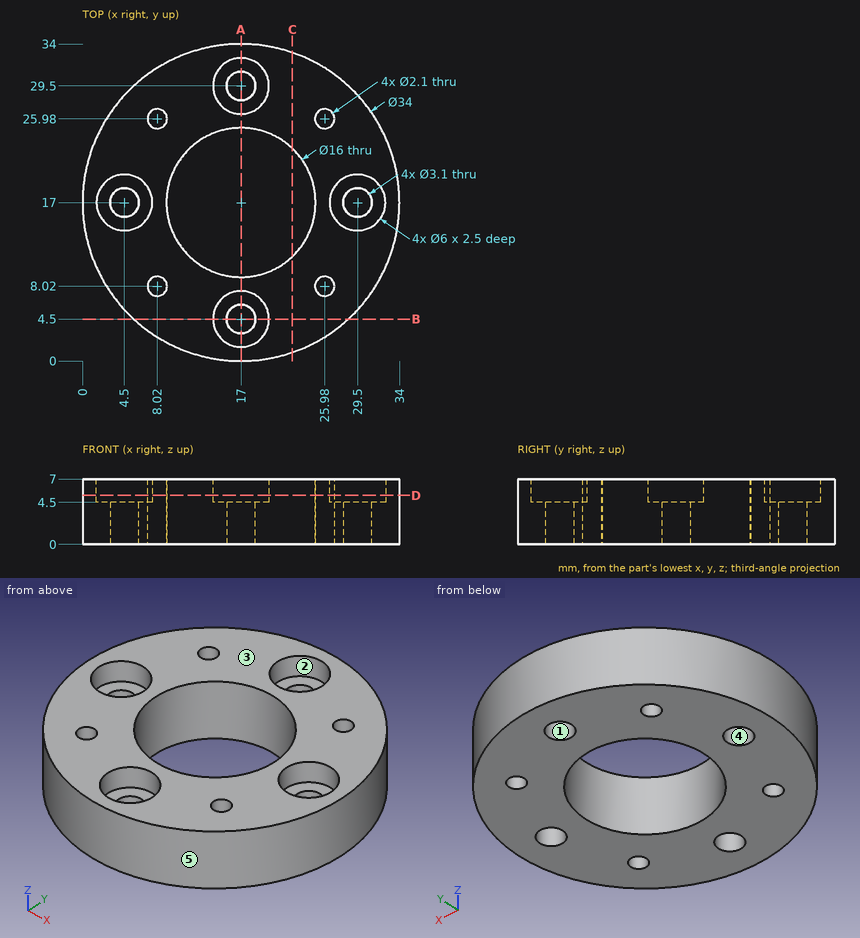
Answer from the drawing. Dimensions are ordinates in mm from the lowest x, y and z of the part. A direction names the side the tool comes from. Round coordinates to 2 decimals unless told otherwise and drop trailing zeros. Write each loop counter-clockwise with the first axis right and the second up, starting at its lowest first coordinate (ties: lowest second). Pieces come first, ordered by that corner, then holes.
1. The part is cut by section D-D, the plane z = 5.25. State how many separate pieces and enclosed holes the cut face has, then the cut area to 3 significant figures.
2. The part is cut by section A-A, the plane x = 17. Determine the outline of the cut face in (y, z).
3. Which of the six approach directions +Z, -Z, +X, -X, +Y, -Y give full straight-line access (tool end or side, diameter ignored) to the marked faces 1 and 2?
4. Straight lines are drawn through the part: L1, parallel to Y at x = 17, z = 1.05; L2, parallel to Y at x = 17, z = 5.25; L3, parallel to X at y = 19, z = 2.25. For each, find the intervals that lie inside material, in ascending order.
5. The part is cut by section B-B, the plane y = 4.5. Determine the outline of the cut face in (x, z).
6. Determine the mould class of the marked faces 3, 4 and 5 for opening direction Y: pulls with the +Y half, pulls with the -Y half, needs draft (parallel to the pull), parting line crosses it, or undercut.
7. Given pin 1 Ø12 at (x, y) = (6, 16) entering from -Z; pin 2 Ø1.9 at (x, y) = (25.98, 25.98) entering from +Z; pin 3 Ø4 at (x, y) = (29.5, 17) entering from +Z; pin 4 Ø3 at (x, z) = (23, 4) entering from -Y, each flat-ended and moving along its own axis, determine where each tip first touches the part or whether it passes through.
8. The part is cut by section C-C, the plane x = 22.5. Determine the outline of the cut face in (y, z).
Values:
1. separate pieces: 1
1. enclosed holes: 9
1. area: 580 mm2
2. outline: (0, 0) - (2.95, 0) - (2.95, 4.5) - (1.5, 4.5) - (1.5, 7) - (0, 7) - close; (6.05, 0) - (9, 0) - (9, 7) - (7.5, 7) - (7.5, 4.5) - (6.05, 4.5) - close; (25, 0) - (27.95, 0) - (27.95, 4.5) - (26.5, 4.5) - (26.5, 7) - (25, 7) - close; (31.05, 0) - (34, 0) - (34, 7) - (32.5, 7) - (32.5, 4.5) - (31.05, 4.5) - close
3. face 1: +Z, -Z
3. face 2: +Z
4. L1: y = 0 to 2.95, 6.05 to 9, 25 to 27.95, 31.05 to 34
4. L2: y = 0 to 1.5, 7.5 to 9, 25 to 26.5, 32.5 to 34
4. L3: x = 0.12 to 9.25, 24.75 to 33.88
5. outline: (5.48, 0) - (15.45, 0) - (15.45, 4.5) - (14, 4.5) - (14, 7) - (5.48, 7) - close; (18.55, 0) - (28.52, 0) - (28.52, 7) - (20, 7) - (20, 4.5) - (18.55, 4.5) - close
6. face 3: needs draft
6. face 4: undercut
6. face 5: parting line crosses it
7. pin 1: stops at z = 0
7. pin 2: passes through
7. pin 3: stops at z = 4.5
7. pin 4: stops at y = 0.61
8. outline: (0.91, 0) - (11.19, 0) - (11.19, 7) - (0.91, 7) - close; (22.81, 0) - (33.09, 0) - (33.09, 7) - (22.81, 7) - close
